Autodesk Fusion 360 part; units mm, degrees
sketch "Sketch1" plane through (0, 0, 0) normal (0, 0, 1) x (1, 0, 0)
  line L0 (10.05, -4.5) -> (-10.05, -4.5)
  line L1 (-10.05, -4.5) -> (-10.05, 4.5)
  line L2 (-10.05, 4.5) -> (10.05, 4.5)
  line L3 (10.05, 4.5) -> (10.05, -4.5)
  line L4 (10.05, -4.5) -> (-10.05, 4.5) construction
  line L5 (-10.05, -4.5) -> (10.05, 4.5) construction
  line L6 (12.05, -6.5) -> (-12.05, -6.5)
  line L7 (-12.05, -6.5) -> (-12.05, 6.5)
  line L8 (-12.05, 6.5) -> (12.05, 6.5)
  line L9 (12.05, 6.5) -> (12.05, -6.5)
  line L10 (-10.05, -4.5) -> (-12.05, -4.5)
  line L11 (10.05, -4.5) -> (12.05, -4.5)
  dimension "d1" = -2
  dimension "d2" = 20.1
  dimension "d3" = 9
extrude "Extrude1" add sketch "Sketch1" along normal mid plane 80 contours L1 L2 L3 L7 L8 L9 L10 L11
sketch "Sketch2" plane through (0, 0, 0) normal (1, 0, 0) x (0, 0, -1)
  line L0 (6, -4.5) -> (-6, -4.5)
  line L1 (-6, -4.5) -> (-6, 3.5)
  line L2 (-6, 3.5) -> (6, 3.5)
  line L3 (6, 3.5) -> (6, -4.5)
  line L4 (6, -4.5) -> (-6, 3.5) construction
  line L5 (-6, -4.5) -> (6, 3.5) construction
  line L6 (40, -4.5) -> (-40, -4.5)
  point P0 (0, -0.5)
  dimension "d6" = 12
  dimension "d7" = 8
extrude "Extrude2" cut sketch "Sketch2" along normal through all and the other way through all
chamfer "Chamfer1" distance 2 angle 45 8 edges at (11.05, -4.5, 6) (11.05, -4.5, -6) (-11.05, -4.5, 6) (-11.05, -4.5, -6) (11.05, -4.5, 40) (-11.05, -4.5, 40) (11.05, -4.5, -40) (-11.05, -4.5, -40)
chamfer "Chamfer2" distance 1 angle 45 2 edges at (0, 4.5, 40) (0, 4.5, -40)
chamfer "Chamfer3" distance 2 angle 45 4 edges at (-11.05, 3.5, 6) (-11.05, 3.5, -6) (11.05, 3.5, 6) (11.05, 3.5, -6)
sketch "Sketch3" plane through (0, 0, 0) normal (1, 0, 0) x (0, 0, -1)
  line L0 (39, 4.5) -> (-39, 4.5)
  line L1 (-39, 4.5) -> (39, 4.5)
  circle A0 centre (0, 4.5) radius 0.75
  circle A1 centre (-32, 4.5) radius 0.75
  circle A2 centre (-24, 4.5) radius 0.75
  circle A3 centre (-16, 4.5) radius 0.75
  circle A4 centre (-8, 4.5) radius 0.75
  circle A5 centre (8, 4.5) radius 0.75
  circle A6 centre (16, 4.5) radius 0.75
  circle A7 centre (24, 4.5) radius 0.75
  circle A8 centre (32, 4.5) radius 0.75
  dimension "d12" = 1.5
  dimension "d15" = 8
  dimension "d16" = 0
extrude "Extrude3" add sketch "Sketch3" along normal up to surface (10.05 mm away) and the other way up to surface (10.05 mm away) contours L0 L1 A8 | L0 L1 A1 | L0 L1 A2 | L0 L1 A3 | L0 L1 A4 | L0 L1 A0 | L0 L1 A5 | L0 L1 A6 | L0 L1 A7 picked at (32.0159, 4.2134) picked at (-32.1559, 4.23) picked at (-24.1944, 4.2563) picked at (-16.1861, 4.2927) picked at (-7.7844, 4.1154) picked at (0.2698, 4.0143) picked at (8.2472, 4.2458) picked at (15.875, 4.0018) picked at (23.8056, 4.2563)
Source: CAD feature listing. Evaluate the final solid. Frame: model axes, mm. A direction names the side the tool comes from. Give positions to 0.01 mm unless a question says otherwise; leave off trailing zeros. Loops run counter-clockwise (first coordinate to the right, second up) from the corner with the lowest first, then second, coordinate; pieces in that order, holes last. Notation, with made-up numbers: (-1, -25.5) - (56, -25.5) arc R26 cw to (56, 10.5) - close; hole circle Ø11 at (-2, 79). An arc over 180 degrees is marked (long way). Use CSV: the item, a comma, the result in double quotes.
1) Pin query (flat end, axial travel): P1, Ø2, axis at x = -3.5, z = -4, coming from the -Y side; P2, Ø5, axis at x = -0.5, z = 24.5, coming from the -Y side; P3, Ø7, axis at x = -1.5, z = -36, coming from the -Y side. Return the tip coordinate at first contact, or that it passes through.
Worked out:
P1,"stops at y = 4.5"
P2,"stops at y = 3.75"
P3,"stops at y = 3.94"
2) Cut plane B-B (z = -14.5). Output: boundary loops of the cut face in (x, y), and give its area (3 significant figures).
Worked out:
outline,"(-12.05, -4.5) - (-10.05, -4.5) - (-10.05, 4.5) - (10.05, 4.5) - (10.05, -4.5) - (12.05, -4.5) - (12.05, 6.5) - (-12.05, 6.5) - close"
area,"84.2 mm^2"
3) Set-up query: faces 4 (the flat face through (-11, -3.5, 39)), 5 (the cylindrical face through (-0.14, 3.75, -0.02)), 6 (the flat face through (11, -1, 6)). Return all of +Z, -Z, +X, -X, +Y, -Y with unobstructed straight access to the full face (end or side cutting, diameter ignored); none if empty.
Worked out:
face 4,"+Z, +X, -X, -Y"
face 5,"-Y"
face 6,"+X, -X, -Y"
4) Mould query, pull axis Z, two halves, no side actions, for faces 1 (the flat face through (0, 4.5, -36)), 2 (the flat face through (0, 6, -40)), 3 (the flat face through (0, 4.5, 4)). Classes: +Z half, -Z half, draft (parallel to the pull), parting line (faces both ways), or undercut.
Worked out:
face 1,"draft"
face 2,"-Z half"
face 3,"undercut"
5) Cut plane A-A (y = -0.75). Output: boundary loops of the cut face in (x, z), and give its area (3 significant figures).
Worked out:
outline,"(-12.05, -40) - (-10.05, -40) - (-10.05, -6) - (-12.05, -6) - close; (-12.05, 6) - (-10.05, 6) - (-10.05, 40) - (-12.05, 40) - close; (10.05, -40) - (12.05, -40) - (12.05, -6) - (10.05, -6) - close; (10.05, 6) - (12.05, 6) - (12.05, 40) - (10.05, 40) - close"
area,"272 mm^2"
6) Line query: line 1 (X direction, y = 2.75, z = -10); line 2 (Y direction, x = 3, z = 28); line 3 (Z direction, x = 10.25, y = 2.25). Output: solid intervals per line, ascending.
Worked out:
line 1,"x = -12.05 to -10.05, 10.05 to 12.05"
line 2,"y = 4.5 to 6.5"
line 3,"z = -40 to -5.25, 5.25 to 40"
7) Cut plane C-C (x = 9.25). Output: boundary loops of the cut face in (y, z), and give its area (3 significant figures).
Worked out:
outline,"(4.5, -39) - (5.5, -40) - (6.5, -40) - (6.5, 40) - (5.5, 40) - (4.5, 39) - (4.5, 32.75) arc R0.75 ccw to (4.5, 31.25) - (4.5, 24.75) arc R0.75 ccw to (4.5, 23.25) - (4.5, 16.75) arc R0.75 ccw to (4.5, 15.25) - (4.5, 8.75) arc R0.75 ccw to (4.5, 7.25) - (4.5, 0.75) arc R0.75 ccw to (4.5, -0.75) - (4.5, -7.25) arc R0.75 ccw to (4.5, -8.75) - (4.5, -15.25) arc R0.75 ccw to (4.5, -16.75) - (4.5, -23.25) arc R0.75 ccw to (4.5, -24.75) - (4.5, -31.25) arc R0.75 ccw to (4.5, -32.75) - close"
area,"167 mm^2"
8) Cut plane D-D (y = 2.5). Output: boundary loops of the cut face in (x, z).
Worked out:
outline,"(-12.05, -40) - (-10.05, -40) - (-10.05, -5) - (-12.05, -5) - close; (-12.05, 5) - (-10.05, 5) - (-10.05, 40) - (-12.05, 40) - close; (10.05, -40) - (12.05, -40) - (12.05, -5) - (10.05, -5) - close; (10.05, 5) - (12.05, 5) - (12.05, 40) - (10.05, 40) - close"
